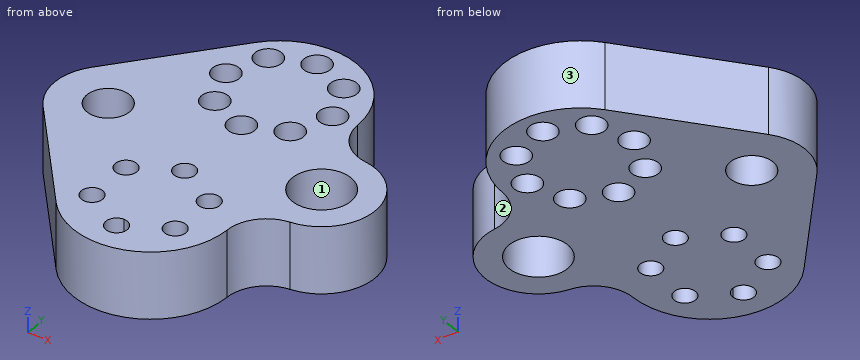
from build123d import *

# Parameters (mm, degrees)
F0_R     = 8
F0_R_2   = 11
F0_R_3   = 4
F0_R_4   = 5
F1_DEPTH = 25


with BuildPart() as f1:
    # F0 (on Top) → F1 (new body)
    with BuildSketch(Plane.XY):
        with BuildLine():
            ThreePointArc((28.995542, 34.508459), (28.998886, 34.254239), (29, 34))
            ThreePointArc((29, 34), (-9.862469, 6.728555), (-22.291842, 52.549226))
            Line((-22.291842, 52.549226), (-55.373684, 12.79257))
            ThreePointArc((-55.373684, 12.79257), (-60, 0), (-55.373684, -12.79257))
            Line((-55.373684, -12.79257), (-22.291842, -52.549226))
            ThreePointArc((-22.291842, -52.549226), (-9.862469, -6.728555), (29, -34))
            ThreePointArc((29, -34), (28.998886, -34.254239), (28.995542, -34.508459))
            ThreePointArc((28.995542, -34.508459), (32.885859, -24.690475), (42.281849, -19.869403))
            ThreePointArc((42.281849, -19.869403), (60, 0), (42.281849, 19.869403))
            ThreePointArc((42.281849, 19.869403), (32.885859, 24.690475), (28.995542, 34.508459))
        make_face()
        with Locations((-40, 0)):
            Circle(F0_R, mode=Mode.SUBTRACT)
        with Locations((40, 0)):
            Circle(F0_R_2, mode=Mode.SUBTRACT)
        with BuildLine():
            ThreePointArc((-22.291842, -52.549226), (9.623005, -61.35686), (28.995542, -34.508459))
            ThreePointArc((28.995542, -34.508459), (28.998886, -34.254239), (29, -34))
            ThreePointArc((29, -34), (-9.862469, -6.728555), (-22.291842, -52.549226))
        make_face()
        with Locations((-15.588457, -43)):
            Circle(F0_R_3, mode=Mode.SUBTRACT)
        with Locations((-15.588457, -25)):
            Circle(F0_R_3, mode=Mode.SUBTRACT)
        with BuildLine():
            ThreePointArc((0, -48), (2.828427, -49.171573), (4, -52))
            ThreePointArc((4, -52), (-2.828427, -54.828427), (0, -48))
        make_face(mode=Mode.SUBTRACT)
        with Locations((15.588457, -43)):
            Circle(F0_R_3, mode=Mode.SUBTRACT)
        with Locations((0, -16)):
            Circle(F0_R_3, mode=Mode.SUBTRACT)
        with Locations((15.588457, -25)):
            Circle(F0_R_3, mode=Mode.SUBTRACT)
        with BuildLine():
            ThreePointArc((-22.291842, 52.549226), (-9.862469, 6.728555), (29, 34))
            ThreePointArc((29, 34), (28.998886, 34.254239), (28.995542, 34.508459))
            ThreePointArc((28.995542, 34.508459), (9.623005, 61.35686), (-22.291842, 52.549226))
        make_face()
        with Locations((-14.142136, 19.857864)):
            Circle(F0_R_4, mode=Mode.SUBTRACT)
        with Locations((-20, 34)):
            Circle(F0_R_4, mode=Mode.SUBTRACT)
        with Locations((-14.142136, 48.142136)):
            Circle(F0_R_4, mode=Mode.SUBTRACT)
        with Locations((0, 14)):
            Circle(F0_R_4, mode=Mode.SUBTRACT)
        with Locations((14.142136, 19.857864)):
            Circle(F0_R_4, mode=Mode.SUBTRACT)
        with Locations((20, 34)):
            Circle(F0_R_4, mode=Mode.SUBTRACT)
        with Locations((0, 54)):
            Circle(F0_R_4, mode=Mode.SUBTRACT)
        with Locations((14.142136, 48.142136)):
            Circle(F0_R_4, mode=Mode.SUBTRACT)
    extrude(amount=F1_DEPTH)


solid = f1.part
Model file for the job. Use its own axes, mm. Face numbers are marked on the shaded views. Coordinates: 2 decimals unless noted, no trailing zeros. Order: outer loops, then holes, each group sorted by start corner. A loop starts at its lowest first (then second) coordinate and runs counter-clockwise, first axis right, second up. Notation, with made-up numbers: (44.25, 36) -> (91.25, 36) arc R28 ccw to (91.25, 64) -> close; hole circle Ø3 at (81, 1.25). An arc over 180 degrees is marked (long way). Return JSON: item names as keys, results as strings. Group by question number.
Item 1: Saw through at D-D on y = -43. Write the cut outline in (x, z), then the cut area to 3 significant figures.
Item 2: Saw through at B-B on x = -40. Write the cut outline in (y, z).
Item 3: Flat gauge pins, fed straight in: P1, Ø21, axis at x = -40, y = 0, coming from the -Z side; P2, Ø2, axis at x = -32, z = 14.5, coming from the -Y side; P3, Ø4, axis at x = -24.5, z = 16, coming from the +Y side; P4, Ø12, axis at x = 4, z = 11, coming from the +Y side. Where does each tip first touch, or does it go through?
Item 4: Saw through at C-C on z = 15.5. State how many separate pieces and enclosed holes the cut face has, then the cut area to 3 significant figures.
Item 5: Pull direction X, two halves, no side cores. Call the marked faces 1, 2 and 3: pulls with the +X half, pulls with the -X half, needs draft (parallel to the pull), parting line crosses it, or undercut.
Item 6: Saw through at A-A on y = -25. Write the cut outline in (x, z), then the cut area to 3 significant figures.
Item 7: Wall check: line 1 along X through (y, z) = (-26, 17); line 2 along Y through (x, z) = (17, 21.5); line 3 along X through (y, z) = (-24.5, 6). Give the ranges that are in metal, low to high. Write a range as [from, to].
Values found:
{
 "1": {"outline": "(-30.24, 0) -> (-19.59, 0) -> (-19.59, 25) -> (-30.24, 25) -> close; (-11.59, 0) -> (11.59, 0) -> (11.59, 25) -> (-11.59, 25) -> close; (19.59, 0) -> (27.57, 0) -> (27.57, 25) -> (19.59, 25) -> close", "area": "1,050 mm2"},
 "2": {"outline": "(-31.27, 0) -> (-8, 0) -> (-8, 25) -> (-31.27, 25) -> close; (8, 0) -> (31.27, 0) -> (31.27, 25) -> (8, 25) -> close"},
 "3": {"P1": "stops at z = 0", "P2": "stops at y = -42.08", "P3": "stops at y = 52.3", "P4": "stops at y = 63"},
 "4": {"separate pieces": "1", "enclosed holes": "16", "area": "7,850 mm2"},
 "5": {"face 1": "undercut", "face 2": "pulls with the +X half", "face 3": "parting line crosses it"},
 "6": {"outline": "(-45.22, 0) -> (-19.59, 0) -> (-19.59, 25) -> (-45.22, 25) -> close; (-11.59, 0) -> (11.59, 0) -> (11.59, 25) -> (-11.59, 25) -> close; (19.59, 0) -> (32.61, 0) -> (32.61, 25) -> (19.59, 25) -> close", "area": "1,550 mm2"},
 "7": {"line 1": "x = [-44.38, -19.46], [-11.72, 11.72], [19.46, 31.83]", "line 2": "y = [-57.49, -46.74], [-39.26, -28.74], [-21.26, 15.76], [23.96, 30], [38, 44.04], [52.24, 57.49]", "line 3": "x = [-45.63, -19.56], [-11.62, 11.62], [19.56, 33.06]"}
}
